Answer from the drawing. Dimensions are ordinates in mm from the lowest x, y and z of the part. Give positions to 0.01 mm unless a question says otherwise; leave off trailing zeros. Write each loop counter-clockwise with the first axis right and the second up, starting at its lowest first coordinate (ties: lowest second). Pieces come first, ordered by that corner, then holes. Notation, with made-up numbers: (-25, -15) -> (-19, -15) arc R30 cw to (-19, 14) -> close; hole circle Ø8 at (15.25, 82.5). An arc over 180 degrees is marked (long way). Use a Markdown table: item, result. Add a question column.
Q1. This flat-tipped pin is pushed along its axis until it touches: pin 1 Ø12 at (x, y) = (31, 68.5) entering from -Z. Where does it stop, or does it pass through?
Q2. Consider line 1 (Y direction, x = 35, z = 7.75); line 2 (Y direction, x = 65.5, z = 4.25); line 3 (X direction, y = 30, z = 2). Determine where each line is inside the solid, lowest interval first.
Q3. Section A-A, the plane z = 3.25 is taken. Give the vertices of the cut face in (x, y), plus the area to 3 significant figures.
Q4. Section B-B, the plane x = 56 is taken. Give the vertices of the cut face in (y, z), plus the area to 3 significant figures.
Q5. Section C-C, the plane y = 52 is taken. Give the vertices of the cut face in (x, z).
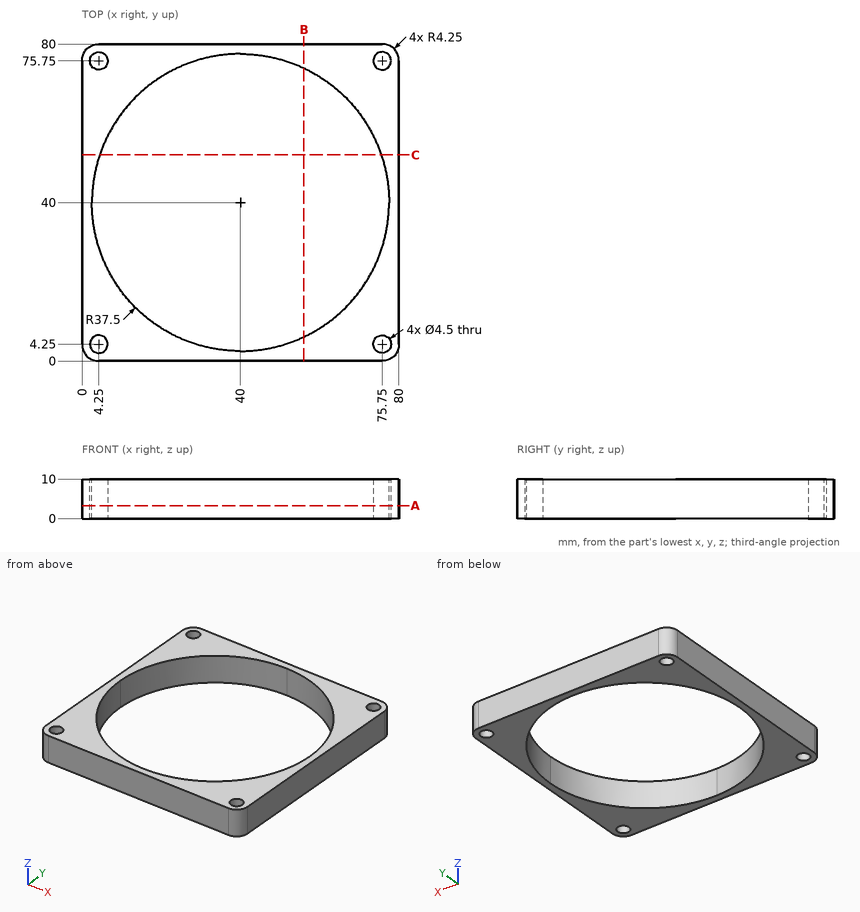
Result set:
| question | item | result |
|---|---|---|
| 1 | pin 1 | passes through |
| 2 | line 1 | y = 0 to 2.83, 77.17 to 80 |
| 2 | line 2 | y = 0 to 12.5, 67.5 to 80 |
| 2 | line 3 | x = 0 to 3.86, 76.14 to 80 |
| 3 | outline | (0, 4.25) arc R4.25 ccw to (4.25, 0) -> (75.75, 0) arc R4.25 ccw to (80, 4.25) -> (80, 75.75) arc R4.25 ccw to (75.75, 80) -> (4.25, 80) arc R4.25 ccw to (0, 75.75) -> close; hole circle Ø4.5 at (4.25, 4.25); hole circle Ø4.5 at (4.25, 75.75); hole (2.5, 40) arc R37.5 ccw to (40, 2.5) arc R37.5 ccw to (77.5, 40) arc R37.5 ccw to (40, 77.5) arc R37.5 ccw to start; hole circle Ø4.5 at (75.75, 4.25); hole circle Ø4.5 at (75.75, 75.75) |
| 3 | area | 1,900 mm2 |
| 4 | outline | (0, 0) -> (6.08, 0) -> (6.08, 10) -> (0, 10) -> close; (73.92, 0) -> (80, 0) -> (80, 10) -> (73.92, 10) -> close |
| 4 | area | 122 mm2 |
| 5 | outline | (0, 0) -> (4.47, 0) -> (4.47, 10) -> (0, 10) -> close; (75.53, 0) -> (80, 0) -> (80, 10) -> (75.53, 10) -> close |
